Build history of the part. All positions in model axes, mm. Round coordinates to 2 decimals unless told otherwise and drop trailing zeros. Write each loop counter-clockwise with the first axis right and the second up, starting at its lowest first coordinate (ties: lowest second). Pieces come first, ordered by that corner, then holes. Notation, with made-up numbers: (25.5, 31.5) -> (34.5, 31.5) arc R28 ccw to (34.5, 56.5) -> close; hole circle Ø7 at (-37, 48). An arc over 180 degrees is marked (long way). Answer as CSV lines item,"result".
from build123d import *

# Parameters (mm, degrees)
SKETCH1_W           = 3
SKETCH1_H           = 3
BOSS_EXTRUDE1_DEPTH = 32.59
SKETCH2_R           = 0.5
CUT_EXTRUDE1_DEPTH  = 4
CUT_EXTRUDE2_REACH  = 5
SKETCH3_R           = 0.500716242


with BuildPart() as part:
    # Sketch1 → Boss-Extrude1 (new body)
    with BuildSketch(Plane(origin=(0, 0, 0), x_dir=(1, 0, 0), z_dir=(0, 1, 0))):
        Rectangle(SKETCH1_W, SKETCH1_H)
    extrude(amount=BOSS_EXTRUDE1_DEPTH)

    # Sketch2 → Cut-Extrude1 (cut, through all)
    with BuildSketch(Plane.XY.offset(1.5)):
        with Locations((0, 1)):
            Circle(SKETCH2_R)
    extrude(amount=-CUT_EXTRUDE1_DEPTH, mode=Mode.SUBTRACT)

    # Sketch3 → Cut-Extrude2 (cut, up to next)
    with BuildSketch(Plane.XY.offset(1.5), mode=Mode.PRIVATE) as cut_extrude2_sk1:
        with Locations((0, 31.59)):
            Circle(SKETCH3_R)
    cut_extrude2_tool1 = extrude(cut_extrude2_sk1.sketch, amount=-CUT_EXTRUDE2_REACH, mode=Mode.PRIVATE) & part.part
    add(cut_extrude2_tool1.solids().sort_by_distance((0, 31.59, 1.5))[0], mode=Mode.SUBTRACT)


solid = part.part
1. Drop a flat-ended pin along its axis: pin 1 Ø1.2 at (x, y) = (0, 31.59) entering from +Z. Give the stop position or say it passes through.
Results found:
pin 1,"stops at z = 1.5"
2. Probe line 1 along Y through (x, z) = (0, 0.75); line 2 along Y through (x, z) = (0.4, -0.35). List the from-to ranges inside material, lowest first.
Results found:
line 1,"y = 0 to 0.5, 1.5 to 31.09, 32.09 to 32.59"
line 2,"y = 0 to 0.7, 1.3 to 31.29, 31.89 to 32.59"
3. Cut at A-A, the plane y = 1. Write the cut outline in (x, z), then the cut area to 3 significant figures.
Results found:
outline,"(-1.5, -1.5) -> (-0.5, -1.5) -> (-0.5, 1.5) -> (-1.5, 1.5) -> close; (0.5, -1.5) -> (1.5, -1.5) -> (1.5, 1.5) -> (0.5, 1.5) -> close"
area,"6.00 mm2"
4. Cut at C-C, the plane z = 0.35. Write the cut outline in (x, y).
Results found:
outline,"(-1.5, 0) -> (1.5, 0) -> (1.5, 32.59) -> (-1.5, 32.59) -> close; hole circle Ø1 at (0, 1); hole circle Ø1 at (0, 31.59)"
5. Cut at B-B, the plane x = 0. Write the cut outline in (y, z).
Results found:
outline,"(0, -1.5) -> (0.5, -1.5) -> (0.5, 1.5) -> (0, 1.5) -> close; (1.5, -1.5) -> (31.09, -1.5) -> (31.09, 1.5) -> (1.5, 1.5) -> close; (32.09, -1.5) -> (32.59, -1.5) -> (32.59, 1.5) -> (32.09, 1.5) -> close"
6. Mould opens along X. For faces 1 (the cylindrical face through (-0.065, 32.086, 0.021)), 2 (the flat face through (0, 0, 0)), 3 (the flat face through (1.5, 16, 0)), 4 (the cylindrical face through (-0.108, 0.512, 0.021)) say: +X half, -X half, draft (parallel to the pull), parting line (faces both ways), or undercut.
Results found:
face 1,"undercut"
face 2,"draft"
face 3,"+X half"
face 4,"undercut"
